from build123d import *

# Parameters (mm, degrees)
SKETCH_1_W          = 73
SKETCH_1_H          = 21
SKETCH_1_R          = 1.05
EXTRUDE_1_DEPTH     = 14
SKETCH_2_W          = 30
SKETCH_2_H          = 15
CUT_EXTRUDE_1_DEPTH = 2


with BuildPart() as part:
    # 草图1 → 凸台-拉伸1 (new body)
    with BuildSketch(Plane(origin=(0, 0, 0), x_dir=(1, 0, 0), z_dir=(0, 1, 0))):
        Rectangle(SKETCH_1_W, SKETCH_1_H)
        with Locations(Location((-20.25, 8.75, 0), (0, 0, 270))):
            Circle(SKETCH_1_R, mode=Mode.SUBTRACT)
        with Locations(Location((20.25, 8.75, 0), (0, 0, 270))):
            Circle(SKETCH_1_R, mode=Mode.SUBTRACT)
        with Locations(Location((20.25, -8.75, 0), (0, 0, 270))):
            Circle(SKETCH_1_R, mode=Mode.SUBTRACT)
        with Locations(Location((-20.25, -8.75, 0), (0, 0, 270))):
            Circle(SKETCH_1_R, mode=Mode.SUBTRACT)
    extrude(amount=EXTRUDE_1_DEPTH)

    # 草图2 → 切除-拉伸1 (cut)
    with BuildSketch(Plane(origin=(0, 14, 0), x_dir=(1, 0, 0), z_dir=(0, 1, 0))):
        with Locations((-1.75, -0.45)):
            Rectangle(SKETCH_2_W, SKETCH_2_H)
    extrude(amount=-CUT_EXTRUDE_1_DEPTH, mode=Mode.SUBTRACT)


solid = part.part
CAD build for the part. Positions are in the model's coordinates, mm. A direction names the side the tool comes from. Coordinates: 2 decimals unless noted, no trailing zeros. Loops run counter-clockwise (first coordinate to the right, second up) from the corner with the lowest first, then second, coordinate; pieces in that order, holes last. Notation, with made-up numbers: (32.5, 86.5) - (88.5, 86.5) arc R20 cw to (88.5, 96.5) - close; hole circle Ø5 at (42.25, 76.25). An arc over 180 degrees is marked (long way). Write item = value, one per line. Start each with the question number.
Q1. Cut at D-D, the plane z = 7. List the corners of the cut face in (x, y).
Q2. Drill centre lines: L1, parallel to X at y = 3.5, z = -8.75; L2, parallel to X at y = 13, z = -1; L3, parallel to X at y = 6, z = 8. Where is each one in solid material? Low to high.
Q3. Pull direction X, two halves, no side cores. Call faces 1 (the flat face through (-1, 7, 10.5)), 2 (the flat face through (-36.5, 7, 0)), 3 (the flat face through (-16.75, 13, 1)): pulls with the +X half, pulls with the -X half, needs draft (parallel to the pull), parting line crosses it, or undercut.
Q4. Cut at B-B, the plane x = -9. List the corners of the cut face in (y, z), then the cut area to 3 significant figures.
Q5. Cut at A-A, the plane z = -8.75. List the corners of the cut face in (x, y).
Q6. Which spindle directions (+Z, -Z, +X, -X, +Y, -Y) get a long thin tool onto all of the face, cutting with end or side? Do faces 4 (the flat face through (-1, 7, -10.5)), 5 (the flat face through (-2, 12, 0)). Say none if no direction does.
Q7. Cut at C-C, the plane x = -20.25. List the corners of the cut face in (y, z), then the cut area to 3 significant figures.
Q8. Flat gauge pins, fed straight in: pin 1 Ø1.9 at (x, z) = (-20.25, -8.75) entering from -Y; pin 2 Ø4.5 at (x, z) = (-5.5, 3.5) entering from +Y. Where does each tip first touch, or does it go through?
Computed:
q1.outline = (-36.5, 0) - (36.5, 0) - (36.5, 14) - (13.25, 14) - (13.25, 12) - (-16.75, 12) - (-16.75, 14) - (-36.5, 14) - close
q2.L1 = -36.5 to -21.3, -19.2 to 19.2, 21.3 to 36.5
q2.L2 = -36.5 to -16.75, 13.25 to 36.5
q2.L3 = -36.5 to -20.98, -19.52 to 19.52, 20.98 to 36.5
q3.face_1 = needs draft
q3.face_2 = pulls with the -X half
q3.face_3 = undercut
q4.outline = (0, -10.5) - (14, -10.5) - (14, -7.05) - (12, -7.05) - (12, 7.95) - (14, 7.95) - (14, 10.5) - (0, 10.5) - close
q4.area = 264 mm²
q5.outline = (-36.5, 0) - (-21.3, 0) - (-21.3, 14) - (-36.5, 14) - close; (-19.2, 0) - (19.2, 0) - (19.2, 14) - (-19.2, 14) - close; (21.3, 0) - (36.5, 0) - (36.5, 14) - (21.3, 14) - close
q6.face_4 = -Z, +X, -X, +Y, -Y
q6.face_5 = +Y
q7.outline = (0, -10.5) - (14, -10.5) - (14, -9.8) - (0, -9.8) - close; (0, -7.7) - (14, -7.7) - (14, 7.7) - (0, 7.7) - close; (0, 9.8) - (14, 9.8) - (14, 10.5) - (0, 10.5) - close
q7.area = 235 mm²
q8.pin_1 = through
q8.pin_2 = 12
